from build123d import *

# Parameters (mm, degrees)
SKETCH1_W               = 76
SKETCH1_H               = 42
SKETCH1_W_2             = 72
SKETCH1_H_2             = 38
BOSS_EXTRUDE1_DEPTH     = 8
SKETCH2_W               = 76
SKETCH2_H               = 42
BOSS_EXTRUDE2_DEPTH     = 1.5
BOSS_EXTRUDE3_START     = -2.4
BOSS_EXTRUDE3_DEPTH     = 7.1
SKETCH4_R               = 1.6
CUT_EXTRUDE1_DEPTH      = 10
SKETCH6_W               = 26
SKETCH6_H               = 2
BOSS_EXTRUDE4_DEPTH     = 16.5
CHAMFER1_SIZE           = 3
CHAMFER2_SIZE           = 3
CUT_EXTRUDE2_DEPTH      = 64.217877218
CUT_EXTRUDE2_DEPTH_BACK = 64.217877218
SKETCH7_R               = 1.6
CHAMFER3_SIZE           = 3


with BuildPart() as part:
    # Sketch1 → Boss-Extrude1 (new body)
    with BuildSketch(Plane(origin=(0, 0, 0), x_dir=(1, 0, 0), z_dir=(0, 1, 0))):
        Rectangle(SKETCH1_W, SKETCH1_H)
        Rectangle(SKETCH1_W_2, SKETCH1_H_2, mode=Mode.SUBTRACT)
    extrude(amount=BOSS_EXTRUDE1_DEPTH)

    # Sketch2 → Boss-Extrude2 (add)
    with BuildSketch(Plane.XZ):
        Rectangle(SKETCH2_W, SKETCH2_H)
    extrude(amount=BOSS_EXTRUDE2_DEPTH)

    # Sketch3 → Boss-Extrude3 (add)
    with BuildSketch(Plane(origin=(0, 8, 0), x_dir=(1, 0, 0), z_dir=(0, 1, 0)).offset(BOSS_EXTRUDE3_START)):
        Polygon((-36, 19), (-36, 16.5), (-34.35, 16.5), (-30.5, 16.5), (30.5, 16.5), (34.35, 16.5), (36, 16.5), (36, 19), align=None)
        with BuildLine():
            Line((-34.35, 16.5), (-36, 16.5))
            Line((-36, 16.5), (-36, -19))
            Line((-36, -19), (-34.35, -19))
            Line((-34.35, -19), (-34.35, 12))
            Line((-34.35, 12), (-34.35, 13.240065792))
            ThreePointArc((-34.35, 13.240065792), (-34.5, 14), (-34.35, 14.759934208))
            Line((-34.35, 14.759934208), (-34.35, 16.5))
        make_face()
        with BuildLine():
            Line((-30.5, 16.5), (-34.35, 16.5))
            Line((-34.35, 16.5), (-34.35, 14.759934208))
            ThreePointArc((-34.35, 14.759934208), (-32.112701665, 15.962141687), (-30.5, 14))
            Line((-30.5, 14), (-30.5, 16.5))
        make_face()
        with BuildLine():
            ThreePointArc((-32.5, 12), (-33.613582414, 12.338695029), (-34.35, 13.240065792))
            Line((-34.35, 13.240065792), (-34.35, 12))
            Line((-34.35, 12), (-32.5, 12))
        make_face()
        with BuildLine():
            ThreePointArc((-30.5, 14), (-32.112701665, 15.962141687), (-34.35, 14.759934208))
            Line((-34.35, 14.759934208), (-34.35, 13.240065792))
            ThreePointArc((-34.35, 13.240065792), (-33.613582414, 12.338695029), (-32.5, 12))
            ThreePointArc((-32.5, 12), (-31.085786438, 12.585786438), (-30.5, 14))
        make_face()
        with BuildLine():
            Line((-34.35, 13.240065792), (-34.35, 14.759934208))
            ThreePointArc((-34.35, 14.759934208), (-34.5, 14), (-34.35, 13.240065792))
        make_face()
        with BuildLine():
            ThreePointArc((34.35, 14.759934208), (32.112701665, 15.962141687), (30.5, 14))
            ThreePointArc((30.5, 14), (31.085786438, 12.585786438), (32.5, 12))
            ThreePointArc((32.5, 12), (33.613582414, 12.338695029), (34.35, 13.240065792))
            Line((34.35, 13.240065792), (34.35, 14.759934208))
        make_face()
        with BuildLine():
            ThreePointArc((34.5, 14), (34.462141687, 14.387298335), (34.35, 14.759934208))
            Line((34.35, 14.759934208), (34.35, 13.240065792))
            ThreePointArc((34.35, 13.240065792), (34.462141687, 13.612701665), (34.5, 14))
        make_face()
        with BuildLine():
            Line((34.35, 16.5), (30.5, 16.5))
            Line((30.5, 16.5), (30.5, 14))
            ThreePointArc((30.5, 14), (32.112701665, 15.962141687), (34.35, 14.759934208))
            Line((34.35, 14.759934208), (34.35, 16.5))
        make_face()
        with BuildLine():
            Line((36, -19), (36, 16.5))
            Line((36, 16.5), (34.35, 16.5))
            Line((34.35, 16.5), (34.35, 14.759934208))
            ThreePointArc((34.35, 14.759934208), (34.462141687, 14.387298335), (34.5, 14))
            ThreePointArc((34.5, 14), (34.462141687, 13.612701665), (34.35, 13.240065792))
            Line((34.35, 13.240065792), (34.35, 12))
            Line((34.35, 12), (34.35, -19))
            Line((34.35, -19), (36, -19))
        make_face()
    extrude(amount=-BOSS_EXTRUDE3_DEPTH)

    # Sketch4 → Cut-Extrude1 (cut)
    with BuildSketch(Plane(origin=(0, 5.6, 0), x_dir=(1, 0, 0), z_dir=(0, 1, 0))):
        with Locations(Location((32.5, 14, 0), (0, 0, 270))):
            Circle(SKETCH4_R)
        with Locations(Location((-32.5, 14, 0), (0, 0, 270))):
            Circle(SKETCH4_R)
    extrude(amount=-CUT_EXTRUDE1_DEPTH, mode=Mode.SUBTRACT)

    # Sketch6 → Boss-Extrude4 (add)
    with BuildSketch(Plane(origin=(0, 0, -21), x_dir=(-1, 0, 0), z_dir=(0, 0, -1))):
        with Locations((37, 7)):
            Rectangle(SKETCH6_W, SKETCH6_H)
    extrude(amount=BOSS_EXTRUDE4_DEPTH)

    # Chamfer1
    chamfer1_edges = [part.edges().sort_by_distance(p)[0] for p in [
        (-31, 6, -21),
    ]]
    chamfer(chamfer1_edges, length=CHAMFER1_SIZE)

    # Chamfer2
    chamfer2_edges = [part.edges().sort_by_distance(p)[0] for p in [
        (-24, 5.5, -21),
        (-24, 7, -37.5),
        (-50, 7, -37.5),
        (-50, 7, -21),
    ]]
    chamfer(chamfer2_edges, length=CHAMFER2_SIZE)

    # Sketch7 → Cut-Extrude2 (cut, two sides: drawn at the far end of the back side and taken through both)
    with BuildSketch(Plane(origin=(0, 8, 0), x_dir=(1, 0, 0), z_dir=(0, 1, 0)).offset(-CUT_EXTRUDE2_DEPTH_BACK)):
        with Locations(Location((-30.5, 33.96, 0), (0, 0, 270))):
            Circle(SKETCH7_R)
        with Locations(Location((-45.8, 33.96, 0), (0, 0, 270))):
            Circle(SKETCH7_R)
    extrude(amount=CUT_EXTRUDE2_DEPTH + CUT_EXTRUDE2_DEPTH_BACK, mode=Mode.SUBTRACT)

    # Chamfer3
    chamfer3_edges = [part.edges().sort_by_distance(p)[0] for p in [
        (-38, 7, -21),
    ]]
    chamfer(chamfer3_edges, length=CHAMFER3_SIZE)


solid = part.part
Geometry: final body of the model. Coordinates: model frame, mm. A direction names the side the tool comes from. Give positions to 0.01 mm unless a question says otherwise; leave off trailing zeros. Loops run counter-clockwise (first coordinate to the right, second up) from the corner with the lowest first, then second, coordinate; pieces in that order, holes last. Notation, with made-up numbers: M 13.5,-33.75 L 20.5,-33.75 A14 cw 20.5,-9.75 Z; hole C 75,-27 d3. An arc over 180 degrees is marked long. Put each result on its own line as item: value. Start each with the question number.
1) Ray query, line 1 along X through (y, z) = (7.5, -33.96); line 2 along Z through (x, y) = (-30.5, 6.7); line 3 along X through (y, z) = (2.5, -14). Return the intervals inside material, ascending.
2) Cut plane D-D (x = 18). Output: boundary loops of the cut face in (y, z), then the cut area to 3 significant figures.
3) Contact query for flat-ended pins moving along their axis: pin 1 (3 mm diameter, centred on x = -45.8, z = -33.96, fed in from -Y); pin 2 (11.5 mm diameter, centred on x = 11, z = 6.5, fed in from +Y); pin 3 (3 mm diameter, centred on y = 1.5, z = -15, fed in from -X); pin 4 (4 mm diameter, centred on x = 6.5, y = 5.5, fed in from -Z). Output: stop coordinate, or through.
4) Cut plane A-A (x = -45.8). Output: boundary loops of the cut face in (y, z), then the cut area to 3 significant figures.
5) Cut plane B-B (y = 4). Output: boundary loops of the cut face in (x, z), then the cut area to 3 significant figures.
6) Cut plane C-C (z = 8). Output: boundary loops of the cut face in (x, y), then the cut area to 3 significant figures.
7) Pull-direction query (Z, two-part tool) for faces 1 (the flat face through (0, 3, -16.5)), 2 (the flat face through (-44, 7, -21)), 3 (the flat face through (-29, 4, -22)); classes: pulls with the +Z half, pulls with the -Z half, needs draft (parallel to the pull), parting line crosses it, or undercut.
8) Access query for faces 4 (the flat face through (-22, 8, -21)), 5 (the flat face through (-34.35, 3, 4)). Directions: +Z, -Z, +X, -X, +Y, -Y. A direction counts if a zero-diameter tool reaches every point of the face in a straight line with its end or side. Return the directions, or none.
Verdict:
1. line 1: -50 to -47.4, -44.2 to -32.1, -28.9 to -24
1. line 2: -37.5 to -35.56, -32.36 to -19, 19 to 21
1. line 3: -38 to -34.1, -30.9 to -30.5, 30.5 to 30.9, 34.1 to 38
2. outline: M -1.5,-21 L 8,-21 L 8,-19 L 5.6,-19 L 5.6,-16.5 L 0,-16.5 L 0,19 L 8,19 L 8,21 L -1.5,21 Z
2. area: 109 mm2
3. pin 1: through
3. pin 2: y = 0
3. pin 3: x = -38
3. pin 4: z = -21
4. outline: M 6,-37.5 L 8,-37.5 L 8,-35.56 L 6,-35.56 Z; M 6,-32.36 L 8,-32.36 L 8,-21 L 6,-21 Z
4. area: 26.6 mm2
5. outline: M -38,-22 L -22,-22 L -21,-21 L 38,-21 L 38,21 L -38,21 Z; hole M -34.35,-12 L -32.5,-12 A2 cw -30.5,-14 L -30.5,-16.5 L 30.5,-16.5 L 30.5,-14 A2 cw 34.35,-13.24 L 34.35,19 L -34.35,19 Z; hole C -32.5,-14 d3.2; hole C 32.5,-14 d3.2
5. area: 786 mm2
6. outline: M -38,-1.5 L 38,-1.5 L 38,8 L 36,8 L 36,5.6 L 34.35,5.6 L 34.35,0 L -34.35,0 L -34.35,5.6 L -36,5.6 L -36,8 L -38,8 Z
6. area: 164 mm2
7. face 1: undercut
7. face 2: pulls with the +Z half
7. face 3: pulls with the -Z half
8. face 4: +Z, -Z, +X, -X, +Y
8. face 5: +Y
